Autodesk Inventor part; units mm, degrees
ref_plane "YZ Plane" through (0, 0, 0) normal (1, 0, 0) x (0, 1, 0)
ref_plane "XZ Plane" through (0, 0, 0) normal (0, 1, 0) x (-1, 0, 0)
ref_plane "XY Plane" through (0, 0, 0) normal (0, 0, 1) x (1, 0, 0)
sketch "Sketch1" plane through (0, 0, 0) normal (0, 0, 1) x (1, 0, 0)
  line L0 (-50, 50) -> (50, 50)
  line L1 (50, 50) -> (50, -50)
  line L2 (50, -50) -> (-50, -50)
  line L3 (-50, -50) -> (-50, 50)
  line L4 (0, 0) -> (0, 5.8013) construction
  line L5 (0, 0) -> (4.5076, 0) construction
  dimension "d0" = 100
  dimension "d1" = 100
extrude "Extrusion1" add sketch "Sketch1" along normal blind 10
sketch "Sketch2" plane through (50, -50, 0) normal (1, 0, 0) x (0, 0, -1)
  line L0 (-10, 100) -> (-10, 0)
  line L1 (-10, 80) -> (-20, 85.7735)
  line L2 (-20, 85.7735) -> (-20, 14.2265)
  line L3 (-20, 14.2265) -> (-10, 20)
  line L4 (0, 100) -> (-10, 100)
  line L5 (0, 0) -> (-10, 0)
  point P0 (0, 50)
  dimension "d4" = 60
  dimension "d5" = 60
  dimension "d6" = 10
  dimension "d7" = 20
  dimension "d8" = 20
extrude "Extrusion2" add sketch "Sketch2" against normal up to surface (100 mm away)
sketch "Sketch3" plane through (0, 0, 0) normal (0, 0, -1) x (-1, 0, 0)
  line L0 (50, -50) -> (50, 50)
  line L1 (50, 50) -> (-50, 50)
  line L2 (-50, -50) -> (50, -50)
  line L3 (-50, 50) -> (-50, -50)
  point P0 (0, 0)
  point P1 (45, -40)
  point P2 (45, 40)
  point P3 (-45, 40)
  point P4 (-45, -40)
  dimension "d11" = 5
  dimension "d12" = 10
  dimension "d13" = 5
  dimension "d14" = 10
  dimension "d15" = 10
  dimension "d16" = 5
  dimension "d17" = 10
  dimension "d18" = 5
hole "Hole1" at (-45, -40, 0) at (-45, 40, 0) at (45, 40, 0) at (45, -40, 0) direction (0, 0, 1) diameter 3.2 end through all
sketch "Sketch4" plane through (-50, 50, 0) normal (0, 1, 0) x (1, 0, 0)
  circle A0 centre (51, -4.6715) radius 1.6
  circle A1 centre (61, -4.6715) radius 1.6
  point P0 (50, 0)
hole "Hole2" at (1, 50, 4.6715) at (11, 50, 4.6715) direction (0, -1, 0) diameter 2.459 depth 13 tip angle 118
properties part number "3d_LM-Welding_Tooling - Moving base" material "Aluminium 6061-T6"
Geometry: final body of the model. Coordinates: model frame, mm. A direction names the side the tool comes from. Round coordinates to 2 decimals unless told otherwise and drop trailing zeros. Loops run counter-clockwise (first coordinate to the right, second up) from the corner with the lowest first, then second, coordinate; pieces in that order, holes last. Notation, with made-up numbers: (43.5, 9.25) -> (66.5, 9.25) arc R13 cw to (66.5, 34.25) -> close; hole circle Ø10 at (56.25, 18). An arc over 180 degrees is marked (long way). Use one line per item in the form item = value.
Item 1: Cut plane D-D on z = 17.25. Output: boundary loops of the cut face in (x, y), then the cut area to 3 significant figures.
Evaluation:
outline = (-50, -34.19) -> (50, -34.19) -> (50, 34.19) -> (-50, 34.19) -> close
area = 6,840 mm2
Item 2: Access query for faces 1 (the flat face through (-1, -40, 10)), 2 (the cylindrical face through (-43.58, 40.74, 5.07)), 3 (the cylindrical face through (0.631, 43.409, 5.844)). Directions: +Z, -Z, +X, -X, +Y, -Y. A direction counts if a zero-diameter tool reaches every point of the face in a straight line with its end or side. Return the directions, or none.
Evaluation:
face_1 = +X, -X, -Y
face_2 = +Z, -Z
face_3 = +Y
Item 3: Contact query for flat-ended pins moving along their axis: pin 1 Ø1.9 at (x, y) = (-45, 40) entering from +Z; pin 2 Ø4 at (x, y) = (45, -40) entering from +Z; pin 3 Ø4 at (x, z) = (17.5, 14.5) entering from -Y. Output: stop coordinate, or through.
Evaluation:
pin_1 = through
pin_2 = 10
pin_3 = -33.75
Item 4: Cut plane C-C on x = -15. Output: boundary loops of the cut face in (y, z), then the cut area to 3 significant figures.
Evaluation:
outline = (-50, 0) -> (50, 0) -> (50, 10) -> (30, 10) -> (35.77, 20) -> (-35.77, 20) -> (-30, 10) -> (-50, 10) -> close
area = 1,660 mm2
Item 5: Cut plane B-B on x = 45. Output: boundary loops of the cut face in (y, z), then the cut area to 3 significant figures.
Evaluation:
outline = (-50, 0) -> (-41.6, 0) -> (-41.6, 10) -> (-50, 10) -> close; (-38.4, 0) -> (38.4, 0) -> (38.4, 10) -> (30, 10) -> (35.77, 20) -> (-35.77, 20) -> (-30, 10) -> (-38.4, 10) -> close; (41.6, 0) -> (50, 0) -> (50, 10) -> (41.6, 10) -> close
area = 1,590 mm2
Item 6: Draft query along Y for faces 4 (the flat face through (0.7, -32.927, 15.07)), 5 (the flat face through (-1, 40, 10)), 6 (the cylindrical face through (46.42, 40.74, 5.07)). Return one class per face: released by +Y, released by -Y, zero draft, split by the parting line, or undercut.
Evaluation:
face_4 = released by -Y
face_5 = zero draft
face_6 = undercut
Item 7: Material intervals for probe 1 along Y at (x, z) = (-45, 3); probe 2 along X at (y, z) = (-40, 7); probe 3 along X at (y, z) = (40, 4.25) (3 decimals), sorted ascending.
Evaluation:
probe_1 = -50 to -41.6, -38.4 to 38.4, 41.6 to 50
probe_2 = -50 to -46.6, -43.4 to 43.4, 46.6 to 50
probe_3 = -50 to -46.6, -43.4 to -0.155, 2.155 to 9.845, 12.155 to 43.4, 46.6 to 50
Item 8: Cut plane A-A on y = -40. Output: boundary loops of the cut face in (x, z), then the cut area to 3 significant figures.
Evaluation:
outline = (-50, 0) -> (-46.6, 0) -> (-46.6, 10) -> (-50, 10) -> close; (-43.4, 0) -> (43.4, 0) -> (43.4, 10) -> (-43.4, 10) -> close; (46.6, 0) -> (50, 0) -> (50, 10) -> (46.6, 10) -> close
area = 936 mm2
